```python
from build123d import *

# Parameters (mm, degrees)
EXTRUDE_1_DEPTH     = 10
SKETCH_2_R          = 2.5
CUT_EXTRUDE_1_DEPTH = 31.528675045


with BuildPart() as part:
    # Эскиз1 → Бобышка-Вытянуть1 (new body)
    with BuildSketch(Plane(origin=(0, 0, 0), x_dir=(1, 0, 0), z_dir=(0, 1, 0))):
        with BuildLine():
            Line((-14, 0), (-24, 0))
            Line((-24, 0), (-24, 2))
            Line((-24, 2), (-15.874507866, 2))
            ThreePointArc((-15.874507866, 2), (0, 16), (15.874507866, 2))
            Line((15.874507866, 2), (24, 2))
            Line((24, 2), (24, 0))
            Line((24, 0), (14, 0))
            ThreePointArc((14, 0), (0, 14), (-14, 0))
        make_face()
    extrude(amount=EXTRUDE_1_DEPTH)

    # Эскиз2 → Вырез-Вытянуть1 (cut, through all)
    with BuildSketch(Plane.XY):
        with Locations((-19, 5)):
            Circle(SKETCH_2_R)
    cut_extrude_1 = extrude(amount=-CUT_EXTRUDE_1_DEPTH, mode=Mode.SUBTRACT)

    # Зеркальное отражение1: Вырез-Вытянуть1 across plane
    add(cut_extrude_1.mirror(Plane(origin=(0, 0, 0), x_dir=(0, 0, 1), z_dir=(1, 0, 0))), mode=Mode.SUBTRACT)


solid = part.part
```
Geometry: final body of the model. Coordinates: model frame, mm. A direction names the side the tool comes from. Round coordinates to 2 decimals unless told otherwise and drop trailing zeros. Loops run counter-clockwise (first coordinate to the right, second up) from the corner with the lowest first, then second, coordinate; pieces in that order, holes last.
Item 1: Section C-C, the plane z = -12.25. Output: boundary loops of the cut face in (x, y), plus the area to 3 significant figures.
Checked values:
outline: (-10.29, 0) - (-6.78, 0) - (-6.78, 10) - (-10.29, 10) - close; (6.78, 0) - (10.29, 0) - (10.29, 10) - (6.78, 10) - close
area: 70.3 mm2
Item 2: Reachability of faces 4 (the flat face through (22, 5, -2)), 5 (the cylindrical face through (-21.5, 5.1, -1)) from +Z, -Z, +X, -X, +Y, -Y: full face, straight path, thin tool, end or side. Return the list, or none.
Checked values:
face 4: -Z, +X, +Y, -Y
face 5: +Z, -Z
Item 3: Section A-A, the plane y = 5. Output: boundary loops of the cut face in (x, z), plus the area to 3 significant figures.
Checked values:
outline: (-24, -2) - (-21.5, -2) - (-21.5, 0) - (-24, 0) - close; (-16.5, -2) - (-15.87, -2) arc R16 ccw to (15.87, -2) - (16.5, -2) - (16.5, 0) - (14, 0) arc R14 cw to (-14, 0) - (-16.5, 0) - close; (21.5, -2) - (24, -2) - (24, 0) - (21.5, 0) - close
area: 106 mm2
Item 4: Mould query, pull axis Z, two halves, no side actions, for faces 1 (the flat face through (21, 3, 0)), 2 (the flat face through (24, 5, -1)), 3 (the flat face through (-22, 5, -2)). Classes: released by +Z, released by -Z, zero draft, split by the parting line, or undercut.
Checked values:
face 1: released by +Z
face 2: zero draft
face 3: released by -Z
Item 5: Section D-D, the plane z = -1.5. Output: boundary loops of the cut face in (x, y), plus the area to 3 significant figures.
Checked values:
outline: (-24, 0) - (-13.92, 0) - (-13.92, 10) - (-24, 10) - close; (13.92, 0) - (24, 0) - (24, 10) - (13.92, 10) - close; hole circle Ø5 at (-19, 5); hole circle Ø5 at (19, 5)
area: 162 mm2
Item 6: Line query: L1, parallel to Y at x = -19, z = -0.85; L2, parallel to X at y = 4.5, z = -4; L3, parallel to Z at x = -18, y = 9. Output: solid intervals per line, ascending.
Checked values:
L1: y = 0 to 2.5, 7.5 to 10
L2: x = -15.49 to -13.42, 13.42 to 15.49
L3: z = -2 to 0
Item 7: Section B-B, the plane x = -19. Output: boundary loops of the cut face in (y, z).
Checked values:
outline: (0, -2) - (2.5, -2) - (2.5, 0) - (0, 0) - close; (7.5, -2) - (10, -2) - (10, 0) - (7.5, 0) - close
Item 8: Contact query for flat-ended pins moving along their axis: P1, Ø6, axis at x = -12.5, z = -2.5, coming from the +Y side; P2, Ø1, axis at y = 6.5, z = -3, coming from the -X side; P3, Ø2.5, axis at x = 21, y = 5, coming from the -Z side. Output: stop coordinate, or through.
Checked values:
P1: stops at y = 10
P2: stops at x = -15.8
P3: stops at z = -2
